```python
from build123d import *

# Parameters (mm, degrees)
SKETCH1_R                        = 55
SKETCH1_R_2                      = 50
BOSS_EXTRUDE1_DEPTH              = 40
SKETCH1_2_R                      = 50
SKETCH1_2_R_2                    = 10
BOSS_EXTRUDE2_DEPTH              = 5
SKETCH1_4_R                      = 28
SKETCH1_4_R_2                    = 25
BOSS_EXTRUDE8_DEPTH              = 20
BOSS_EXTRUDE8_DRAFT              = 1
SKETCH2_R                        = 4.5
BOSS_EXTRUDE3_DEPTH              = 35
FILLET1_R                        = 6
CIRPATTERN1_COUNT                = 3
FILLET1_OF_CIRPATTERN1_R         = 6
BOSS_EXTRUDE7_DEPTH              = 40
FILLET2_R                        = 12
F_5_0MM_DOWEL_HOLE1_D            = 5
F_5_0MM_DOWEL_HOLE1_CSINK_D      = 5.05
F_5_0MM_DOWEL_HOLE1_CSINK_ANGLE  = 90
F_12_0MM_DOWEL_HOLE1_D           = 12
F_12_0MM_DOWEL_HOLE1_CSINK_D     = 12.05
F_12_0MM_DOWEL_HOLE1_CSINK_ANGLE = 90
FILLET3_R                        = 12
CIRPATTERN2_COUNT                = 2
FILLET2_OF_CIRPATTERN2_R         = 12
FILLET3_OF_CIRPATTERN2_R         = 12


with BuildPart() as part:
    # Sketch1 → Boss-Extrude1 (new body)
    with BuildSketch(Plane(origin=(0, 0, 0), x_dir=(1, 0, 0), z_dir=(0, 1, 0))):
        with Locations(Location((0, 0, 0), (0, 0, 270))):
            Circle(SKETCH1_R)
        with Locations(Location((0, 0, 0), (0, 0, 270))):
            Circle(SKETCH1_R_2, mode=Mode.SUBTRACT)
    extrude(amount=BOSS_EXTRUDE1_DEPTH)

    # Sketch1<2> → Boss-Extrude2 (add)
    with BuildSketch(Plane(origin=(0, 0, 0), x_dir=(1, 0, 0), z_dir=(0, 1, 0))):
        with Locations(Location((0, 0, 0), (0, 0, 270))):
            Circle(SKETCH1_2_R)
        with Locations(Location((0, 0, 0), (0, 0, 270))):
            Circle(SKETCH1_2_R_2, mode=Mode.SUBTRACT)
    extrude(amount=BOSS_EXTRUDE2_DEPTH)


with BuildPart() as boss_extrude8_tool:
    # Sketch1<4> → Boss-Extrude8 (with draft: the straight prism first)
    with BuildSketch(Plane(origin=(0, 0, 0), x_dir=(1, 0, 0), z_dir=(0, 1, 0))):
        Circle(SKETCH1_4_R)
        Circle(SKETCH1_4_R_2, mode=Mode.SUBTRACT)
    extrude(amount=BOSS_EXTRUDE8_DEPTH)
    # Boss-Extrude8: the draft: its side faces are tilted about the plane it starts from
    boss_extrude8_sides = [boss_extrude8_tool.faces().sort_by_distance(p)[0] for p in [
        (-28, 10, 0),
        (-25, 10, 0),
    ]]
    draft(boss_extrude8_sides, Plane(origin=(0, 0, 0), x_dir=(1, 0, 0), z_dir=(0, 1, 0)), BOSS_EXTRUDE8_DRAFT)


with BuildPart() as part_1:
    add(part.part)

    # Boss-Extrude8: add boss_extrude8_tool
    add(boss_extrude8_tool.part)

    # Sketch2 → Boss-Extrude3 (add)
    with BuildSketch(Plane(origin=(0, 5, 0), x_dir=(1, 0, 0), z_dir=(0, 1, 0))):
        with BuildLine():
            ThreePointArc((-12.220451707, 48.483611252), (0, 37.685826265), (12.220451707, 48.483611252))
            ThreePointArc((12.220451707, 48.483611252), (0, 50), (-12.220451707, 48.483611252))
        make_face()
        with Locations(Location((0, 44.925923132, 0), (0, 0, 270))):
            Circle(SKETCH2_R, mode=Mode.SUBTRACT)
    boss_extrude3 = extrude(amount=BOSS_EXTRUDE3_DEPTH)

    # Fillet1
    fillet1_edges = [part_1.edges().sort_by_distance(p)[0] for p in [
        (12.220451707, 22.5, -48.483611252),
        (-12.220451707, 22.5, -48.483611252),
    ]]
    fillet(fillet1_edges, radius=FILLET1_R)

    # CirPattern1: Boss-Extrude3 ×3 about axis
    cirpattern1_axis = Axis((0, 0, 0), (0, 1, 0))
    for i in range(1, CIRPATTERN1_COUNT):
        add(boss_extrude3.rotate(cirpattern1_axis, i * 360 / CIRPATTERN1_COUNT))

    # Fillet1 of CirPattern1
    fillet1_of_cirpattern1_edges = [part_1.edges().sort_by_distance(p)[0] for p in [
        (-48.098264865, 22.5, 13.658584002),
        (-35.877813158, 22.5, 34.825027251),
        (35.877813158, 22.5, 34.825027251),
        (48.098264865, 22.5, 13.658584002),
    ]]
    fillet(fillet1_of_cirpattern1_edges, radius=FILLET1_OF_CIRPATTERN1_R)

    # Sketch3 → Boss-Extrude7 (add)
    with BuildSketch(Plane.XZ):
        with BuildLine():
            Line((0, -55), (0, -85))
            Line((0, -85), (-10, -85))
            Line((-10, -85), (-10, -54.083269132))
            ThreePointArc((-10, -54.083269132), (-5.02096593, -54.770337785), (0, -55))
        make_face()
    boss_extrude7 = extrude(amount=-BOSS_EXTRUDE7_DEPTH)

    # Fillet2
    fillet2_edges = [part_1.edges().sort_by_distance(p)[0] for p in [
        (-10, 20, -54.083269132),
    ]]
    fillet(fillet2_edges, radius=FILLET2_R)

    # Ø5.0mm Dowel Hole1 (through all)
    with Locations(Plane(origin=(0, 0, 0), x_dir=(0, 0, -1), z_dir=(1, 0, 0))):
        with Locations((70, 32), (70, 8)):
            f_5_0mm_dowel_hole1 = CounterSinkHole(F_5_0MM_DOWEL_HOLE1_D / 2, F_5_0MM_DOWEL_HOLE1_CSINK_D / 2, counter_sink_angle=F_5_0MM_DOWEL_HOLE1_CSINK_ANGLE)

    # Ø12.0mm Dowel Hole1 (through all)
    with Locations(Plane(origin=(0, 0, 0), x_dir=(0, 0, -1), z_dir=(1, 0, 0))):
        with Locations((70, 20)):
            f_12_0mm_dowel_hole1 = CounterSinkHole(F_12_0MM_DOWEL_HOLE1_D / 2, F_12_0MM_DOWEL_HOLE1_CSINK_D / 2, counter_sink_angle=F_12_0MM_DOWEL_HOLE1_CSINK_ANGLE)

    # Fillet3
    fillet3_edges = [part_1.edges().sort_by_distance(p)[0] for p in [
        (-5, 0, -85),
        (-5, 40, -85),
    ]]
    fillet(fillet3_edges, radius=FILLET3_R)

    # CirPattern2: Boss-Extrude7, Ø5.0mm Dowel Hole1, Ø12.0mm Dowel Hole1 ×2 about axis
    cirpattern2_axis = Axis((0, 0, 0), (0, 1, 0))
    add([boss_extrude7.rotate(cirpattern2_axis, i * 360 / CIRPATTERN2_COUNT) for i in range(1, CIRPATTERN2_COUNT)])
    add([f_5_0mm_dowel_hole1.rotate(cirpattern2_axis, i * 360 / CIRPATTERN2_COUNT) for i in range(1, CIRPATTERN2_COUNT)], mode=Mode.SUBTRACT)
    add([f_12_0mm_dowel_hole1.rotate(cirpattern2_axis, i * 360 / CIRPATTERN2_COUNT) for i in range(1, CIRPATTERN2_COUNT)], mode=Mode.SUBTRACT)

    # Fillet2 of CirPattern2
    fillet2_of_cirpattern2_edges = [part_1.edges().sort_by_distance(p)[0] for p in [
        (10, 20, 54.083269132),
    ]]
    fillet(fillet2_of_cirpattern2_edges, radius=FILLET2_OF_CIRPATTERN2_R)

    # Fillet3 of CirPattern2
    fillet3_of_cirpattern2_edges = [part_1.edges().sort_by_distance(p)[0] for p in [
        (5, 0, 85),
        (5, 40, 85),
    ]]
    fillet(fillet3_of_cirpattern2_edges, radius=FILLET3_OF_CIRPATTERN2_R)


solid = part_1.part
```
Geometry check sheet. Reference: the model listing, model coordinates, mm. A direction names the side the tool comes from. Coordinates: 2 decimals unless noted, no trailing zeros. Order: outer loops, then holes, each group sorted by start corner. A loop starts at its lowest first (then second) coordinate and runs counter-clockwise, first axis right, second up. Notation, with made-up numbers: (-25, 7.5) - (9, 7.5) arc R20 cw to (9, 46.5) - close; hole circle Ø11 at (-33.5, 58). An arc over 180 degrees is marked (long way). Answer as a JSON object with one key per item and string values. Group by question number.
Item 1: Depth check by flat-ended pin: pin 1 Ø10 at (y, z) = (29.5, 49) entering from -X; pin 2 Ø8 at (x, y) = (24, 6) entering from -Z; pin 3 Ø1.5 at (y, z) = (16.5, -25.5) entering from -X. Enter the tip coordinate at first touch or a pass-through.
Item 2: Sectioned sample at A-A, the plane z = -70. Record the cut outline in (x, y) (3 decimals), and give its area (3 significant figures).
Item 3: Draft check along X on faces 4 (the face through (5.08, 33.69, 71.84)), 5 (the face through (54.4, 19.7, -8.1)), 6 (the face through (12.2, 20, 22.4)). Enter one of: +X half, -X half, draft (parallel to the pull), parting line (faces both ways), or undercut.
Item 4: Sectioned sample at B-B, the plane y = 32. Give the number of separate pieces and of enclosed holes in the cut face, and give its area (3 significant figures).
Item 5: Tool access check on faces 1 (the face through (0, 20, -63)), 2 (the face through (10, 20, 77)), 3 (the face through (-32.55, 22.26, 19)). Record the directions out of +Z, -Z, +X, -X, +Y, -Y that give a thin tool (end or side, any length) a straight path to the whole face; none if there is none.
Item 6: Scan lines: probe 1 along Y at (x, z) = (6.5, 70); probe 2 along Z at (x, y) = (33, 26.5); probe 3 along Y at (x, z) = (15.5, 29.5). Record each from-to range of solid material in increasing order.
Resolved:
{
 "1": {"pin 1": "x = -33", "pin 2": "z = -51.23", "pin 3": "x = -49.12"},
 "2": {"outline": "(-10, 0) - (0, 0) - (0, 5.475) - (-0.025, 5.5) - (-10, 5.5) - close; (-10, 10.5) - (-0.025, 10.5) - (0, 10.525) - (0, 13.975) - (-0.025, 14) - (-10, 14) - close; (-10, 26) - (-0.025, 26) - (0, 26.025) - (0, 29.475) - (-0.025, 29.5) - (-10, 29.5) - close; (-10, 34.5) - (-0.025, 34.5) - (0, 34.525) - (0, 40) - (-10, 40) - close", "area": "180 mm^2"},
 "3": {"face 4": "draft", "face 5": "+X half", "face 6": "undercut"},
 "4": {"separate pieces": "3", "enclosed holes": "4", "area": "2,700 mm^2"},
 "5": {"face 1": "-Z, +X, +Y, -Y", "face 2": "+Z, +X, +Y, -Y", "face 3": "+Y"},
 "6": {"probe 1": "0 to 5.5, 10.5 to 14, 26 to 29.5, 34.5 to 40", "probe 2": "-44 to -37.56, 18.25 to 31.84, 36.8 to 44", "probe 3": "0 to 5"}
}
